Design review of the part built by this model. Coordinates are the model's own, in mm. A direction names the side the tool comes from. Round coordinates to 2 decimals unless told otherwise and drop trailing zeros. Order: outer loops, then holes, each group sorted by start corner. A loop starts at its lowest first (then second) coordinate and runs counter-clockwise, first axis right, second up.
from build123d import *

# Parameters (mm, degrees)
SKETCH1_W           = 53
SKETCH1_H           = 105.8
BOSS_EXTRUDE1_DEPTH = 5


with BuildPart() as part:
    # Sketch1 → Boss-Extrude1 (new body)
    with BuildSketch(Plane.XY):
        Polygon((127.9, 63.9), (-55.082401894, 63.9), (-55.082401894, 51.9), (-3.5, 51.9), (-3.5, -53.9), (-55.082401894, -53.9), (-55.082401894, -73.9), (127.9, -73.9), (127.9, 51.9), align=None)
        with Locations((30, -1)):
            Rectangle(SKETCH1_W, SKETCH1_H, mode=Mode.SUBTRACT)
        Polygon((113.412674799, 51.9), (63.5, 51.9), (63.5, 23.082903769), align=None, mode=Mode.SUBTRACT)
        Polygon((113.412674799, -53.9), (63.5, -53.9), (63.5, -25.082903769), align=None, mode=Mode.SUBTRACT)
        Polygon((117.9, 46.407854644), (117.9, -48.407854644), (63.5, -17), (63.5, 15), align=None, mode=Mode.SUBTRACT)
    extrude(amount=BOSS_EXTRUDE1_DEPTH)


solid = part.part
1) The part is to be moulded in two halves that separate along Y. For faces 4 (the face through (3.5, -2, 2)), 5 (the face through (38, 63.9, 2)), 6 (the face through (-55.082, 58, 2)), say which applies: released by +Y, released by -Y, zero draft, split by the parting line, or undercut.
Results:
face 4: undercut
face 5: released by +Y
face 6: zero draft
2) To check wall thickness, follow line 1 along X through (y, z) = (5, 3.9); line 2 along X through (y, z) = (-50, 2.45); line 3 along Y through (x, z) = (-4.5, 1.6). State the ranges of each line that lie inside material, in increasing order.
Results:
line 1: x = -3.5 to 3.5, 56.5 to 63.5, 117.9 to 127.9
line 2: x = -3.5 to 3.5, 56.5 to 63.5, 106.66 to 127.9
line 3: y = -73.9 to -53.9, 51.9 to 63.9
3) Take a section at A-A on y = -3.5. Give the boundary of the cut face in (x, z), plus the area to 3 significant figures.
Results:
outline: (-3.5, 0) - (3.5, 0) - (3.5, 5) - (-3.5, 5) - close; (56.5, 0) - (63.5, 0) - (63.5, 5) - (56.5, 5) - close; (117.9, 0) - (127.9, 0) - (127.9, 5) - (117.9, 5) - close
area: 120 mm2
4) For faces 1 (the face through (63, -15, 5)), 2 (the face through (-3.5, 0, 2)), 3 (the face through (89, 51.9, 2)), list the 3-axis set-ups (+Z, -Z, +X, -X, +Y, -Y) from which the entire face can be reached by the end or side of a thin tool; tool diameter is ignored.
Results:
face 1: +Z, +X, -X, +Y, -Y
face 2: +Z, -Z, -X
face 3: +Z, -Z
5) Take a section at C-C on x = -19.5. Give the boundary of the cut face in (y, z).
Results:
outline: (-73.9, 0) - (-53.9, 0) - (-53.9, 5) - (-73.9, 5) - close; (51.9, 0) - (63.9, 0) - (63.9, 5) - (51.9, 5) - close
6) Take a section at B-B on z = 3.05. Give the boundary of the cut face in (x, y), plus the area to 3 significant figures.
Results:
outline: (-55.08, -73.9) - (127.9, -73.9) - (127.9, 63.9) - (-55.08, 63.9) - (-55.08, 51.9) - (-3.5, 51.9) - (-3.5, -53.9) - (-55.08, -53.9) - close; hole (3.5, -53.9) - (56.5, -53.9) - (56.5, 51.9) - (3.5, 51.9) - close; hole (63.5, -53.9) - (113.41, -53.9) - (63.5, -25.08) - close; hole (63.5, -17) - (117.9, -48.41) - (117.9, 46.41) - (63.5, 15) - close; hole (63.5, 23.08) - (113.41, 51.9) - (63.5, 51.9) - close
area: 9,260 mm2
7) Clearance check with flat-ended pins moving along their axes: P1, Ø2, axis at x = 18, y = -53.5, coming from the -Z side; P2, Ø2, axis at y = 43.5, z = 4, coming from the -X side. State where each tip first meets the part, or that it passes through.
Results:
P1: stops at z = 0
P2: stops at x = -3.5
8) Take a section at D-D on x = 102. Give the boundary of the cut face in (y, z), plus the area to 3 significant figures.
Results:
outline: (-73.9, 0) - (-53.9, 0) - (-53.9, 5) - (-73.9, 5) - close; (-47.31, 0) - (-39.23, 0) - (-39.23, 5) - (-47.31, 5) - close; (37.23, 0) - (45.31, 0) - (45.31, 5) - (37.23, 5) - close; (51.9, 0) - (63.9, 0) - (63.9, 5) - (51.9, 5) - close
area: 241 mm2
